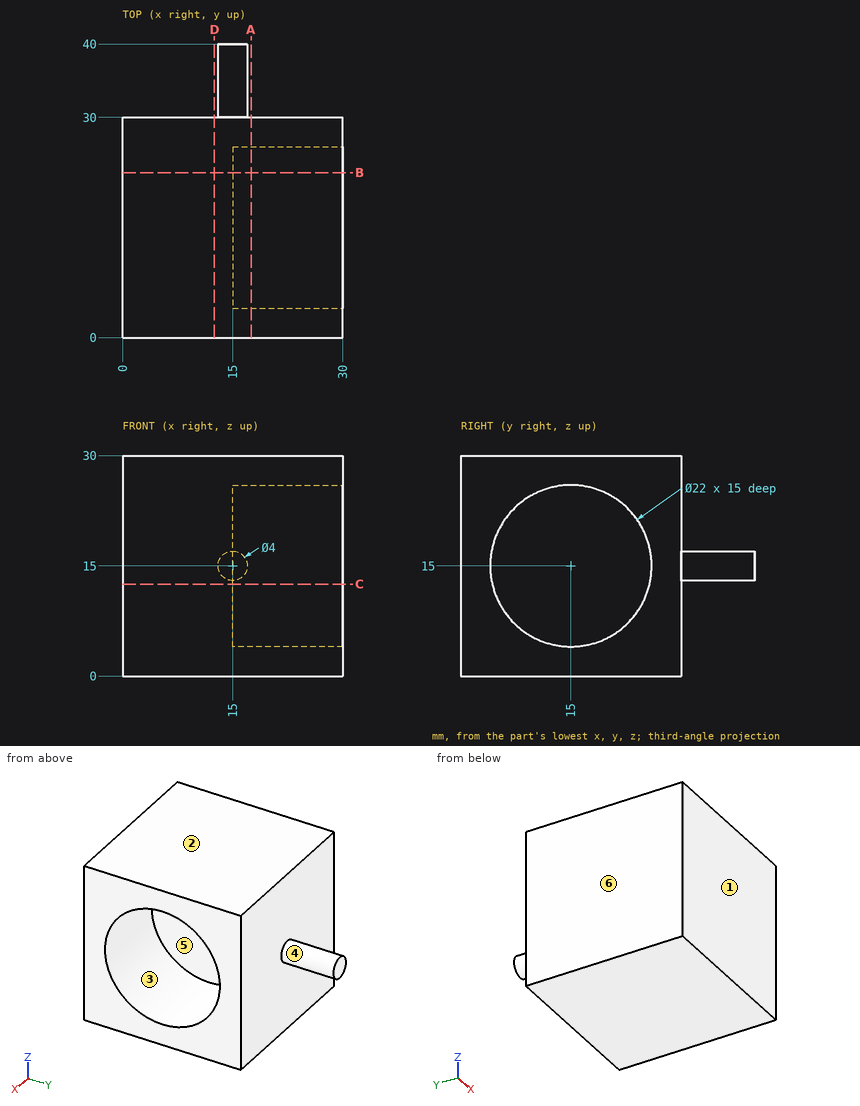
Print and shaded views of the part. All mm, measured from the part's lowest x, y and z. A direction names the side the tool comes from. Coordinates: 2 decimals unless noted, no trailing zeros. Order: outer loops, then holes, each group sorted by start corner. A loop starts at its lowest first (then second) coordinate and runs counter-clockwise, first axis right, second up. Notation, with made-up numbers: M -30.5,-27 L 14.5,-27 A23 cw 14.5,10 Z; hole C -16,49 d2. An arc over 180 degrees is marked long. Answer as CSV lines item,"result".
1) Cut at C-C (z = 12.5). List the corners of the cut face in (x, y), then the cut area to 3 significant figures.
Verdict:
outline,"M 0,0 L 30,0 L 30,4.29 L 15,4.29 L 15,25.71 L 30,25.71 L 30,30 L 0,30 Z"
area,"579 mm2"
2) Flat gauge pins, fed straight in: P1, Ø1, axis at x = 6, z = 21, coming from the +Y side; P2, Ø1.5, axis at y = 14.5, z = 22.5, coming from the +X side. Where does each tip first touch, or does it go through?
Verdict:
P1,"y = 30"
P2,"x = 15"
3) Mould opens along Z. For the marked faces 1, 2 and 3 say: released by +Z, released by -Z, zero draft, split by the parting line, or undercut.
Verdict:
face 1,"zero draft"
face 2,"released by +Z"
face 3,"undercut"
4) Cut at A-A (x = 17.5). List the corners of the cut face in (y, z).
Verdict:
outline,"M 0,0 L 30,0 L 30,30 L 0,30 Z; hole C 15,15 d22"
5) 3-axis set-ups, long thin cutter, end or side, ignore diameter. For the marked faces 4, 5 and 6: which of +Z, -Z, +X, -X, +Y, -Y reach the whole face in a straight line?
Verdict:
face 4,"+Y"
face 5,"+X"
face 6,"+Z, -Z, -X, +Y, -Y"
6) Cut at D-D (x = 12.5). List the corners of the cut face in (y, z), then the cut area to 3 significant figures.
Verdict:
outline,"M 0,0 L 30,0 L 30,30 L 0,30 Z"
area,"900 mm2"
7) Drill centre lines: L1, parallel to Y at x = 26, z = 15; L2, parallel to X at y = 18.5, z = 20.5; L3, parallel to Y at x = 14, z = 7.5. Where is each one in solid material? Low to high. Write a range as from..to.
Verdict:
L1,"0..4, 26..30"
L2,"0..15"
L3,"0..30"
8) Cut at B-B (y = 22.5). List the corners of the cut face in (x, z), then the cut area to 3 significant figures.
Verdict:
outline,"M 0,0 L 30,0 L 30,6.95 L 15,6.95 L 15,23.05 L 30,23.05 L 30,30 L 0,30 Z"
area,"659 mm2"
